Source: CAD feature listing. Evaluate the final solid. Frame: model axes, mm. A direction names the side the tool comes from. Round coordinates to 2 decimals unless told otherwise and drop trailing zeros. Order: outer loops, then holes, each group sorted by start corner. A loop starts at its lowest first (then second) coordinate and runs counter-clockwise, first axis right, second up. Notation, with made-up numbers: (89, -17.75) -> (122, -17.75) arc R25 cw to (122, -4.75) -> close; hole circle Ø8 at (32.5, 12). An arc over 180 degrees is marked (long way). Use a Markdown table: item, result. Add a question column.
```python
from build123d import *

# Parameters (mm, degrees)
F1_DEPTH = 63.5
F0_W     = 25.4
F0_H     = 19.05
F0_H_2   = 4.7498
F0_H_3   = 4.7752
F2_DEPTH = 25.4
F3_DEPTH = 3.175


with BuildPart() as f1:
    # F0 (on Front) → F1 (new body, symmetric)
    with BuildSketch(Plane.XZ):
        Polygon((41.275, -9.525), (41.275, 9.525), (22.225, 9.525), (-41.275, 9.525), (-41.275, -9.525), align=None)
    extrude(amount=F1_DEPTH, both=True)

    # F0 (on Front) → F2 (join, symmetric)
    with BuildSketch(Plane.XZ):
        with BuildLine():
            Line((22.225, 9.525), (41.275, 9.525))
            Line((41.275, 9.525), (41.275, 27.0002))
            ThreePointArc((41.275, 27.0002), (45.9246798487, 38.2255201513), (57.15, 42.8752))
            Line((57.15, 42.8752), (60.325, 42.8752))
            Line((60.325, 42.8752), (60.325, 61.9252))
            Line((60.325, 61.9252), (57.15, 61.9252))
            ThreePointArc((57.15, 61.9252), (32.4542956671, 51.6959043329), (22.225, 27.0002))
            Line((22.225, 27.0002), (22.225, 9.525))
        make_face()
        with Locations((73.025, 52.4002)):
            Rectangle(F0_W, F0_H)
        with Locations((73.025, 64.3001)):
            Rectangle(F0_W, F0_H_2)
        with Locations((73.025, 40.4876)):
            Rectangle(F0_W, F0_H_3)
    extrude(amount=F2_DEPTH, both=True)

    # F0 (on Front) → F3 (join, symmetric)
    with BuildSketch(Plane.XZ):
        with BuildLine():
            Line((-41.275, 9.525), (22.225, 9.525))
            Line((22.225, 9.525), (22.225, 27.0002))
            ThreePointArc((22.225, 27.0002), (32.4542956671, 51.6959043329), (57.15, 61.9252))
            add(Edge.make_bspline(
                [(-41.275, 9.525), (-40.8707372844, 40.7271385193), (-5.9925662354, 61.9721710682), (57.15, 61.9252)],
                knots=[0, 0, 0, 0, 111.5045361635, 111.5045361635, 111.5045361635, 111.5045361635], degree=3))
        make_face()
    extrude(amount=F3_DEPTH, both=True)


solid = f1.part
```
1) Section C-C on x = 73.5. Output: boundary loops of the cut face in (y, z) (3 decimals).
2) First-contact query: pin 1 Ø1.5 at (x, z) = (10.5, 33.5) entering from -Y (3 decimals); pin 2 Ø14 at (y, z) = (-19, 18.5) entering from -X (3 decimals); pin 3 Ø12 at (x, y) = (-21, 15.5) entering from +Z (3 decimals); pin 4 Ø12 at (y, z) = (-36, 16) entering from -X. Flat tips, straight axial feed; report the tip coordinate or a pass-through.
3) Line query: probe 1 along Z at (x, y) = (26, -48.5) (3 decimals); probe 2 along Y at (x, z) = (-1, 27) (3 decimals); probe 3 along X at (y, z) = (-7.5, 13.5) (3 decimals). Output: solid intervals per line, ascending. Write a range as from..to.
4) Reachability of faces 1 (the flat face through (22.225, 14, 18)), 2 (the flat face through (59, 0, 61.925)), 3 (the flat face through (73, 0, 38.1)) from +Z, -Z, +X, -X, +Y, -Y: full face, straight path, thin tool, end or side. Return the list, or none.
5) Draft query along X for faces 4 (the flat face through (54, -25.4, 45)), 5 (the flat face through (22.225, -14, 18)), 6 (the cylindrical face through (45.8, -0.4, 38.1)). Return one class per face: pulls with the +X half, pulls with the -X half, needs draft (parallel to the pull), parting line crosses it, or undercut.
6) Section A-A on y = -15.5. Output: boundary loops of the cut face in (x, z) (3 decimals).
7) Section B-B on z = 5.5. Output: boundary loops of the cut face in (x, y) (3 decimals), then the cut area to 3 significant figures.
Conclusion:
| question | item | result |
|---|---|---|
| 1 | outline | (-25.4, 38.1) -> (25.4, 38.1) -> (25.4, 66.675) -> (-25.4, 66.675) -> close |
| 2 | pin 1 | stops at y = -3.175 |
| 2 | pin 2 | stops at x = 22.225 |
| 2 | pin 3 | stops at z = 9.525 |
| 2 | pin 4 | passes through |
| 3 | probe 1 | z = -9.525..9.525 |
| 3 | probe 2 | y = -3.175..3.175 |
| 3 | probe 3 | x = 22.225..41.275 |
| 4 | face 1 | +Z, -X, +Y |
| 4 | face 2 | +Z, -X, +Y, -Y |
| 4 | face 3 | -Z, +X, +Y, -Y |
| 5 | face 4 | needs draft |
| 5 | face 5 | pulls with the -X half |
| 5 | face 6 | undercut |
| 6 | outline | (-41.275, -9.525) -> (41.275, -9.525) -> (41.275, 27) arc R15.875 cw to (57.15, 42.875) -> (60.325, 42.875) -> (60.325, 38.1) -> (85.725, 38.1) -> (85.725, 66.675) -> (60.325, 66.675) -> (60.325, 61.925) -> (57.15, 61.925) arc R34.925 ccw to (22.225, 27) -> (22.225, 9.525) -> (-41.275, 9.525) -> close |
| 7 | outline | (-41.275, -63.5) -> (41.275, -63.5) -> (41.275, 63.5) -> (-41.275, 63.5) -> close |
| 7 | area | 10,500 mm^2 |
